Read the model definition and answer for the solid it produces. Units are mm, in the model's axes. Face numbers are marked on the shaded views. A direction names the side the tool comes from. Coordinates: 2 decimals unless noted, no trailing zeros. Loops run counter-clockwise (first coordinate to the right, second up) from the corner with the lowest first, then second, coordinate; pieces in that order, holes last. Notation, with made-up numbers: (77, 34) -> (121, 34) arc R10 ccw to (121, 45) -> close; hole circle Ø11 at (-13, 88.5). An arc over 180 degrees is marked (long way). One line per question, with ' | ' between items. Start each with the question number.
```python
from build123d import *

# Parameters (mm, degrees)
F_70MM_45_3MM_START   = -35
F_70MM_45_3MM_DEPTH   = 70
EXTRUDE_START         = 2
SKETCH_8_W            = 70
SKETCH_8_H            = 8
EXTRUDE_307_DEPTH     = 32
EXTRUDE_START_2       = 3
SKETCH_9_R            = 1.65
EXTRUDE_M3_1_DEPTH    = 3
SKETCH_10_R           = 1.65
EXTRUDE_M3_1_2_DEPTH  = 3
F_36X48_M3_DEPTH      = 3.1
F_36X48_M3_DEPTH_BACK = 3.1
SKETCH_11_R           = 1.65
CUT_EXTRUDE_START     = -8
SKETCH_12_R           = 3.2
CUT_EXTRUDE_818_DEPTH = 3.8


with BuildPart() as part:
    # 草图1 → 70mm紧凑45度雷达承托面_3mm (new body)
    with BuildSketch(Plane(origin=(0, 0, 0), x_dir=(0, 0, -1), z_dir=(1, 0, 0)).offset(F_70MM_45_3MM_START)):
        Polygon((16.748737342, -84.748737342), (-32.748737342, -35.251262658), (-30.627416998, -33.129942315), (18.870057685, -82.627416998), align=None)
    extrude(amount=F_70MM_45_3MM_DEPTH)

    # 草图8 → Extrude 307 (add)
    with BuildSketch(Plane.XY.offset(EXTRUDE_START)):
        with Locations((0, -32)):
            Rectangle(SKETCH_8_W, SKETCH_8_H)
    extrude(amount=EXTRUDE_307_DEPTH)

    # 草图9 → Extrude M3__-1 (add)
    with BuildSketch(Plane.XY.offset(EXTRUDE_START_2)):
        with BuildLine():
            Line((-32, -28), (-26, -28))
            ThreePointArc((-26, -28), (-24.585786438, -27.414213562), (-24, -26))
            Line((-24, -26), (-24, -20))
            ThreePointArc((-24, -20), (-24.585786438, -18.585786438), (-26, -18))
            Line((-26, -18), (-32, -18))
            ThreePointArc((-32, -18), (-33.414213562, -18.585786438), (-34, -20))
            Line((-34, -20), (-34, -26))
            ThreePointArc((-34, -26), (-33.414213562, -27.414213562), (-32, -28))
        make_face()
        with Locations((-29, -23)):
            Circle(SKETCH_9_R, mode=Mode.SUBTRACT)
    extrude(amount=EXTRUDE_M3_1_DEPTH)

    # 草图10 → Extrude M3__1 2 (add)
    with BuildSketch(Plane.XY.offset(EXTRUDE_START_2)):
        with BuildLine():
            Line((26, -28), (32, -28))
            ThreePointArc((32, -28), (33.414213562, -27.414213562), (34, -26))
            Line((34, -26), (34, -20))
            ThreePointArc((34, -20), (33.414213562, -18.585786438), (32, -18))
            Line((32, -18), (26, -18))
            ThreePointArc((26, -18), (24.585786438, -18.585786438), (24, -20))
            Line((24, -20), (24, -26))
            ThreePointArc((24, -26), (24.585786438, -27.414213562), (26, -28))
        make_face()
        with Locations((29, -23)):
            Circle(SKETCH_10_R, mode=Mode.SUBTRACT)
    extrude(amount=EXTRUDE_M3_1_2_DEPTH)

    # 草图11 → 端口朝下雷达36x48四M3孔 (cut, two sides: drawn at the far end of the back side and taken through both)
    with BuildSketch(Plane(origin=(0, -34, 34), x_dir=(1, 0, 0), z_dir=(0, -0.7071067811865477, 0.7071067811865475)).offset(-F_36X48_M3_DEPTH_BACK)):
        with Locations(Location((-18, -60.769552622, 0), (0, 0, 270))):
            Circle(SKETCH_11_R)
        with Locations(Location((-18, -12.769552622, 0), (0, 0, 270))):
            Circle(SKETCH_11_R)
        with Locations(Location((18, -60.769552622, 0), (0, 0, 270))):
            Circle(SKETCH_11_R)
        with Locations(Location((18, -12.769552622, 0), (0, 0, 270))):
            Circle(SKETCH_11_R)
    extrude(amount=F_36X48_M3_DEPTH + F_36X48_M3_DEPTH_BACK, mode=Mode.SUBTRACT)

    # 草图12 → Cut-Extrude 818 (cut)
    with BuildSketch(Plane(origin=(0, -34, 34), x_dir=(1, 0, 0), z_dir=(0, -0.7071067811865477, 0.7071067811865475)).offset(CUT_EXTRUDE_START)):
        with Locations((-18, -12.769552622)):
            Circle(SKETCH_12_R)
        with Locations((18, -12.769552622)):
            Circle(SKETCH_12_R)
    extrude(amount=CUT_EXTRUDE_818_DEPTH, mode=Mode.SUBTRACT)


solid = part.part
```
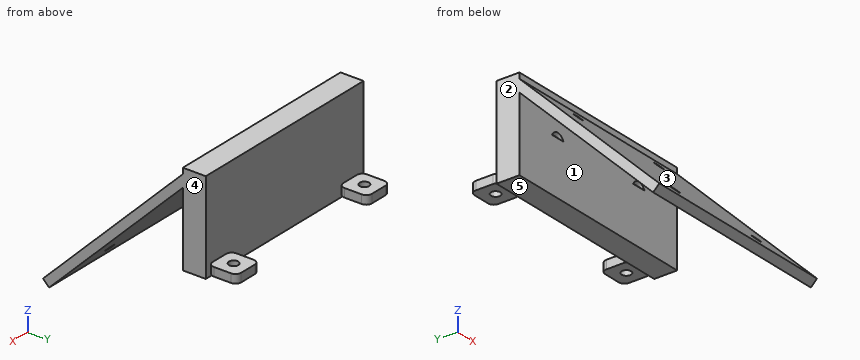
(1) Section C-C on x = -9.5 is taken. Write down the section's boundary in (y, z), plus the area to 3 significant figures.
(2) Determine the mould class of the marked faces 1, 2 and 3 for opening direction Y: +Y half, -Y half, draft (parallel to the pull), parting line (faces both ways), or undercut.
(3) A tool of negligible diameter and unlimited length cuts with its end or side. For the marked faces 4 and 5, from which of +Z, -Z, +X, -X, +Y, -Y can it reach the whole face along a straight path? Write none if from no direction.
(4) Section D-D on z = 16.5 is taken. Write down the section's boundary in (x, y).
(5) Each of these flat-tipped pins is pushed along its axis until it touches: pin 1 Ø3.5 at (y, z) = (-23, 5) entering from +X; pin 2 Ø3 at (x, z) = (26.5, 24.5) entering from -Y; pin 3 Ø1 at (x, y) = (25, -27) entering from -Z. Where does it stop, or does it pass through?
(6) Section B-B on x = -29 is taken. Write down the section's boundary in (y, z).
(7) Section A-A on z = 5 is taken. Write down the section's boundary in (x, y), plus the area to 3 significant figures.
(8) Find the intervals of material crossed by probe 1 along Y at (x, z) = (-29, 4); probe 2 along Y at (x, z) = (-29, 5); probe 3 along Z at (x, y) = (-19, -30), in increasing order. Write a range as from..to.
Working result:
1) outline: (-84.75, -16.75) -> (-82.63, -18.87) -> (-36, 27.76) -> (-36, 2) -> (-28, 2) -> (-28, 34) -> (-36, 34) -> (-36, 32) -> close | area: 458 mm2
2) face 1: undercut | face 2: draft | face 3: -Y half
3) face 4: +Z, -Z, +X, +Y, -Y | face 5: -Z, +X, -X, +Y
4) outline: (-35, -51.5) -> (35, -51.5) -> (35, -47.26) -> (-35, -47.26) -> close; (-35, -36) -> (35, -36) -> (35, -28) -> (-35, -28) -> close
5) pin 1: stops at x = 34 | pin 2: stops at y = -45 | pin 3: stops at z = 3
6) outline: (-84.75, -16.75) -> (-82.63, -18.87) -> (-36, 27.76) -> (-36, 2) -> (-28, 2) -> (-28, 3) -> (-24.65, 3) -> (-24.65, 6) -> (-28, 6) -> (-28, 34) -> (-36, 34) -> (-36, 32) -> close; (-21.35, 3) -> (-18, 3) -> (-18, 6) -> (-21.35, 6) -> close
7) outline: (-35, -63) -> (35, -63) -> (35, -58.76) -> (-35, -58.76) -> close; (-35, -36) -> (35, -36) -> (35, -28) -> (32, -28) arc R2 ccw to (34, -26) -> (34, -20) arc R2 ccw to (32, -18) -> (26, -18) arc R2 ccw to (24, -20) -> (24, -26) arc R2 ccw to (26, -28) -> (-26, -28) arc R2 ccw to (-24, -26) -> (-24, -20) arc R2 ccw to (-26, -18) -> (-32, -18) arc R2 ccw to (-34, -20) -> (-34, -26) arc R2 ccw to (-32, -28) -> (-35, -28) -> close; hole circle Ø3.3 at (-29, -23); hole circle Ø3.3 at (29, -23) | area: 1,030 mm2
8) probe 1: y = -64..-59.76, -36..-24.65, -21.35..-18 | probe 2: y = -63..-58.76, -36..-24.65, -21.35..-18 | probe 3: z = 2..34
